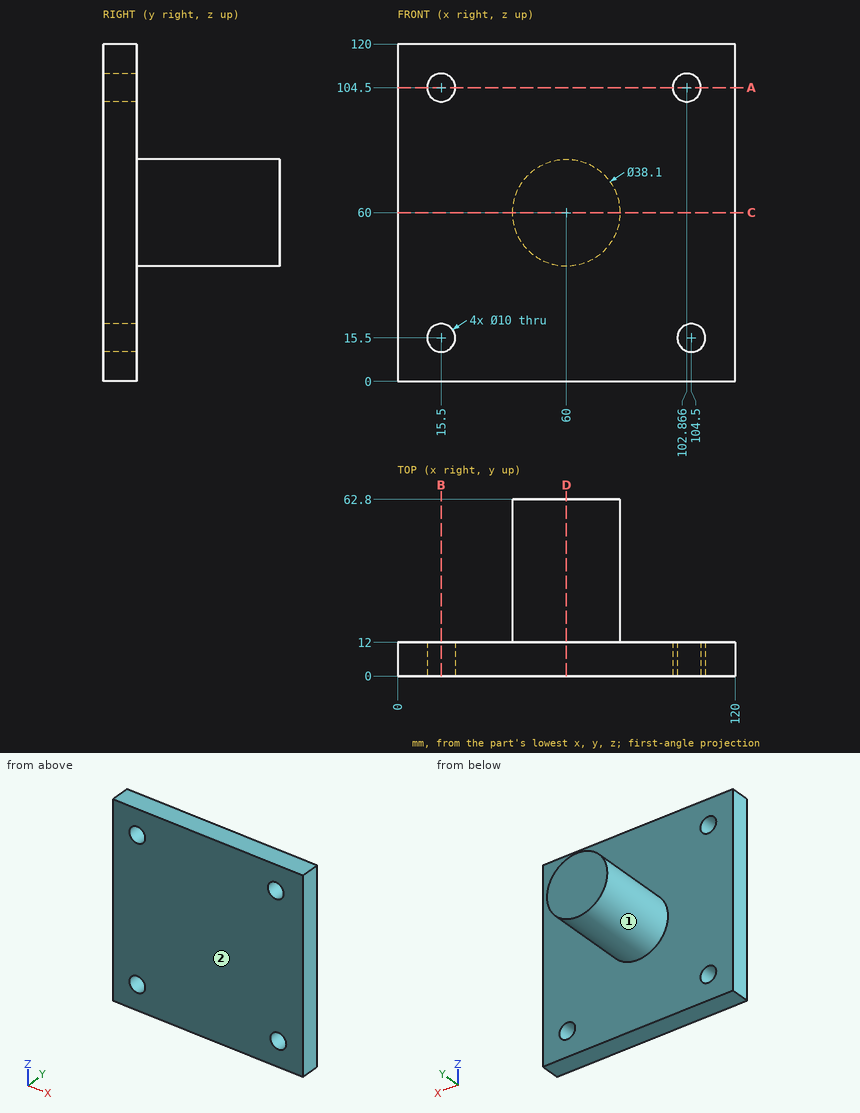
Input: dimensioned drawing with shaded views. Units: mm. Origin: part minimum x, y, z. A direction names the side the tool comes from. Coordinates: 2 decimals unless noted, no trailing zeros. Loops run counter-clockwise (first coordinate to the right, second up) from the corner with the lowest first, then second, coordinate; pieces in that order, holes last. Notation, with made-up numbers: (40, 41) -> (90, 41) arc R16 ccw to (90, 45) -> close; hole circle Ø11 at (-16, 77.25). An arc over 180 degrees is marked (long way). Use a Markdown table: item, result. Add a question column.
(1) Section query B-B, the plane x = 15.5. Return loops of the section in (y, z), plus the area to 3 significant figures.
(2) Section query A-A, the plane z = 104.5. Return loops of the section in (x, y), plus the area to 3 significant figures.
(3) Section query D-D, the plane x = 60. Return loops of the section in (y, z).
(4) Access query for the marked faces 1 and 2. Directions: +Z, -Z, +X, -X, +Y, -Y. A direction counts if a zero-diameter tool reaches every point of the face in a straight line with its end or side. Return the directions, or none.
(5) Line query: line 1 along X through (y, z) = (5.25, 104.5); line 2 along Z through (x, y) = (15.5, 3). Output: solid intervals per line, ascending.
(6) Pin query (flat end, axial travel): pin 1 Ø4 at (x, y) = (75, 28) entering from +Z (1 decimal); pin 2 Ø4 at (y, z) = (20, 54) entering from +X (1 decimal); pin 3 Ø13 at (x, z) = (15.5, 104.5) entering from +Y. Return the tip coordinate at first contact, or that it passes through.
(7) Section query C-C, the plane z = 60. Return loops of the section in (x, y).
Answer:
| question | item | result |
|---|---|---|
| 1 | outline | (0, 0) -> (12, 0) -> (12, 10.5) -> (0, 10.5) -> close; (0, 20.5) -> (12, 20.5) -> (12, 99.5) -> (0, 99.5) -> close; (0, 109.5) -> (12, 109.5) -> (12, 120) -> (0, 120) -> close |
| 1 | area | 1,200 mm^2 |
| 2 | outline | (0, 0) -> (10.5, 0) -> (10.5, 12) -> (0, 12) -> close; (20.5, 0) -> (97.87, 0) -> (97.87, 12) -> (20.5, 12) -> close; (107.87, 0) -> (120, 0) -> (120, 12) -> (107.87, 12) -> close |
| 2 | area | 1,200 mm^2 |
| 3 | outline | (0, 0) -> (12, 0) -> (12, 40.95) -> (62.8, 40.95) -> (62.8, 79.05) -> (12, 79.05) -> (12, 120) -> (0, 120) -> close |
| 4 | face 1 | +Y |
| 4 | face 2 | +Z, -Z, +X, -X, -Y |
| 5 | line 1 | x = 0 to 10.5, 20.5 to 97.87, 107.87 to 120 |
| 5 | line 2 | z = 0 to 10.5, 20.5 to 99.5, 109.5 to 120 |
| 6 | pin 1 | stops at z = 73.9 |
| 6 | pin 2 | stops at x = 78.6 |
| 6 | pin 3 | stops at y = 12 |
| 7 | outline | (0, 0) -> (120, 0) -> (120, 12) -> (79.05, 12) -> (79.05, 62.8) -> (40.95, 62.8) -> (40.95, 12) -> (0, 12) -> close |
